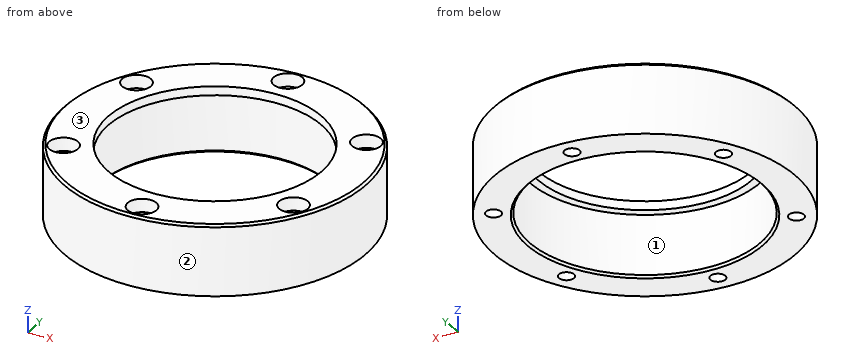
Autodesk Inventor part; units mm, degrees
ref_plane "YZ Plane" through (0, 0, 0) normal (1, 0, 0) x (0, 1, 0)
ref_plane "XZ Plane" through (0, 0, 0) normal (0, 1, 0) x (-1, 0, 0)
ref_plane "XY Plane" through (0, 0, 0) normal (0, 0, 1) x (1, 0, 0)
sketch "スケッチ2" plane through (0, 0, 0) normal (1, 0, 0) x (0, 1, 0)
  line L0 (0, 0) -> (26.1, 0)
  line L1 (26.1, 0) -> (26.1, -16)
  line L2 (26.1, -16) -> (0, -16)
  line L3 (0, -16) -> (0, 0)
  line L4 (0, 0) -> (34.1, 0)
  line L5 (34.1, 0) -> (34.1, -16)
  line L6 (34.1, -16) -> (0, -16)
  line L7 (0, -16) -> (0, 0)
  line L8 (34.1, 0) -> (21, 0)
  line L9 (26.1, 0) -> (24.1, 0)
  line L10 (24.1, 0) -> (24.1, -2)
  line L11 (24.1, -2) -> (26.1, -2)
  line L12 (26.1, -2) -> (26.1, 0)
  point P0 (26.1, 0)
  point P1 (24.1, 0)
  dimension "d1" = 26.1
  dimension "d8" = 2
  dimension "d10" = 14
  dimension "d27" = 8
  dimension "d31" = 2
revolve "回転1" add sketch "スケッチ2" angle 360 about axis through (0, 0, -16) along (0, 0, 1) contours L0 L1 L11 L10 | L1 L4 L5 L6
sketch "スケッチ4" plane through (0, 0, 0) normal (0, 0, 1) x (1, 0, 0)
  point P0 (0, 0)
  point P1 (0, 30)
  point P2 (-25.9808, 15)
  point P3 (-25.9808, -15)
  point P4 (0, -30)
  point P5 (25.9808, -15)
  point P6 (25.9808, 15)
  dimension "d11" = 30
  dimension "d14" = 360
hole "穴1" at (0, 30, 0) at (-25.9808, 15, 0) at (-25.9808, -15, 0) at (0, -30, 0) at (25.9808, -15, 0) at (25.9808, 15, 0) direction (0, 0, -1) diameter 3.4 end through all counterbore diameter 6.5 counterbore depth 3
chamfer "面取り1" distance 0.5 angle 45 1 edges at (0, -26.1, -16)
chamfer "面取り2" distance 0.5 angle 45 1 edges at (0, -34.1, 0)
properties part number "bearing_cover_j5" material "ABS プラスチック"
Geometry check sheet. Reference: the model listing, model coordinates, mm. Face numbers are marked on the shaded views. Give positions to 0.01 mm unless a question says otherwise; leave off trailing zeros. Write each loop counter-clockwise with the first axis right and the second up, starting at its lowest first coordinate (ties: lowest second). Pieces come first, ordered by that corner, then holes. Notation, with made-up numbers: (-40, -21.5) -> (-5, -21.5) arc R22 ccw to (-5, -15.5) -> close; hole circle Ø7 at (79, 36.25). An arc over 180 degrees is marked (long way). Use one line per item in the form item = value.
Item 1: Depth check by flat-ended pin: pin 1 Ø6 at (x, y) = (0, 30) entering from +Z; pin 2 Ø6 at (x, z) = (-17.5, -12.5) entering from -Y; pin 3 Ø2.5 at (x, y) = (25.98, 15) entering from -Z; pin 4 Ø5 at (x, y) = (20.5, -12.5) entering from -Z. Enter the tip coordinate at first touch or a pass-through.
Results list:
pin_1 = -3
pin_2 = -30.86
pin_3 = through
pin_4 = -15.91
Item 2: Sectioned sample at B-B on y = 0. Enter the section's corners in (x, z), plus the area to 4 significant figures.
Results list:
outline = (-34.1, -16) -> (-26.6, -16) -> (-26.1, -15.5) -> (-26.1, -2) -> (-24.1, -2) -> (-24.1, 0) -> (-33.6, 0) -> (-34.1, -0.5) -> close; (24.1, -2) -> (26.1, -2) -> (26.1, -15.5) -> (26.6, -16) -> (34.1, -16) -> (34.1, -0.5) -> (33.6, 0) -> (24.1, 0) -> close
area = 263.5 mm2
Item 3: Sectioned sample at A-A on x = 0. Count the separate pieces of the cut face and the enclosed holes in it, plus the area to 3 significant figures.
Results list:
separate_pieces = 4
enclosed_holes = 0
area = 136 mm2
Item 4: Mould release check, pull along Y, two halves, no side actions. Record for the marked faces 1, 2 and 3: released by +Y, released by -Y, zero draft, split by the parting line, or undercut.
Results list:
face_1 = undercut
face_2 = split by the parting line
face_3 = zero draft
Item 5: Scan lines: line 1 (Y direction, x = 0, z = -5); line 2 (X direction, y = -15, z = -1.55); line 3 (Z direction, x = -24, y = -8.5). Record each from-to range of solid material in increasing order.
Results list:
line_1 = -34.1 to -31.7, -28.3 to -26.1, 26.1 to 28.3, 31.7 to 34.1
line_2 = -30.62 to -29.23, -22.73 to -18.86, 18.86 to 22.73, 29.23 to 30.62
line_3 = -2 to 0
Item 6: Sectioned sample at C-C on z = -10. Enter the section's corners in (x, y).
Results list:
outline = circle Ø68.2 at (0, 0); hole circle Ø3.4 at (-25.98, -15); hole circle Ø3.4 at (-25.98, 15); hole circle Ø52.2 at (0, 0); hole circle Ø3.4 at (0, -30); hole circle Ø3.4 at (0, 30); hole circle Ø3.4 at (25.98, -15); hole circle Ø3.4 at (25.98, 15)
